Geometry: final body of the model. Coordinates: model frame, mm. A direction names the side the tool comes from. Coordinates: 2 decimals unless noted, no trailing zeros. Write each loop counter-clockwise with the first axis right and the second up, starting at its lowest first coordinate (ties: lowest second). Pieces come first, ordered by that corner, then holes.
from build123d import *

# Parameters (mm, degrees)
SKETCH2_W           = 80
SKETCH2_H           = 80
BOSS_EXTRUDE1_DEPTH = 5
BOSS_EXTRUDE2_DEPTH = 1
CUT_EXTRUDE1_DEPTH  = 3


with BuildPart() as part:
    # Sketch2 → Boss-Extrude1 (new body)
    with BuildSketch(Plane(origin=(0, 0, 0), x_dir=(0, 0, -1), z_dir=(1, 0, 0))):
        with Locations((40, 40)):
            Rectangle(SKETCH2_W, SKETCH2_H)
    extrude(amount=BOSS_EXTRUDE1_DEPTH)

    # Sketch3 → Boss-Extrude2 (add)
    with BuildSketch(Plane(origin=(5, 0, 0), x_dir=(0, 0, -1), z_dir=(1, 0, 0))):
        with BuildLine():
            Line((57, 32.75895), (57, 47.24105))
            ThreePointArc((57, 47.24105), (21.522099548, 40), (57, 32.75895))
        make_face()
    extrude(amount=BOSS_EXTRUDE2_DEPTH)

    # Sketch4 → Cut-Extrude1 (cut)
    with BuildSketch(Plane(origin=(6, 0, 0), x_dir=(0, 0, -1), z_dir=(1, 0, 0))):
        with BuildLine():
            Line((57.5, 32.75895), (57.5, 47.24105))
            ThreePointArc((57.5, 47.24105), (21.061076981, 40), (57.5, 32.75895))
        make_face()
    extrude(amount=-CUT_EXTRUDE1_DEPTH, mode=Mode.SUBTRACT)


solid = part.part
Item 1: Section A-A, the plane y = 40. Output: boundary loops of the cut face in (x, z), plus the area to 3 significant figures.
Derived:
outline: (0, -80) - (5, -80) - (5, -57.5) - (3, -57.5) - (3, -21.06) - (5, -21.06) - (5, 0) - (0, 0) - close
area: 327 mm2
Item 2: Material intervals for probe 1 along Y at (x, z) = (3.6, -40); probe 2 along Z at (x, y) = (4.25, 40); probe 3 along X at (y, z) = (44, -25), sorted ascending.
Derived:
probe 1: y = 0 to 21.06, 58.94 to 80
probe 2: z = -80 to -57.5, -21.06 to 0
probe 3: x = 0 to 3
Item 3: Set-up query: faces 1 (the flat face through (5, 49, -57)), 2 (the cylindrical face through (4.014, 40.729, -21.075)). Return all of +Z, -Z, +X, -X, +Y, -Y with unobstructed straight access to the full face (end or side cutting, diameter ignored); none if empty.
Derived:
face 1: +Z, -Z, +X, +Y, -Y
face 2: +X
Item 4: Section B-B, the plane z = -40. Output: boundary loops of the cut face in (x, y).
Derived:
outline: (0, 0) - (5, 0) - (5, 21.06) - (3, 21.06) - (3, 58.94) - (5, 58.94) - (5, 80) - (0, 80) - close
Item 5: Section C-C, the plane x = 4. Output: boundary loops of the cut face in (y, z).
Derived:
outline: (0, -80) - (80, -80) - (80, 0) - (0, 0) - close; hole (32.76, -57.5) - (47.24, -57.5) arc R18.94 ccw (long way) to start
Item 6: Pin query (flat end, axial travel): pin 1 (8 mm diameter, centred on y = 51.5, z = -32, fed in from +X). Return the tip coordinate at first contact, or that it passes through.
Derived:
pin 1: stops at x = 3
Item 7: Pull-direction query (Y, two-part tool) for faces 3 (the flat face through (2, 80, -39)), 4 (the flat face through (4, 40, -57.5)), 5 (the flat face through (0, 41, -39)); classes: released by +Y, released by -Y, zero draft, split by the parting line, or undercut.
Derived:
face 3: released by +Y
face 4: undercut
face 5: zero draft
